Can you work these out from the model? Positions are in its coordinate system, mm. Face numbers are marked on the shaded views. A direction names the side the tool comes from. Round coordinates to 2 decimals unless told otherwise and drop trailing zeros. Order: outer loops, then holes, each group sorted by start corner. A loop starts at its lowest first (then second) coordinate and runs counter-clockwise, first axis right, second up. Notation, with made-up numbers: (68.5, 27) - (91.5, 27) arc R25 ccw to (91.5, 48) - close; hole circle Ø10 at (-22, 30.5). An arc over 180 degrees is marked (long way). Write item = value, one per line.
from build123d import *

# Parameters (mm, degrees)
P_IDAT_VYSUNUT_M1_DEPTH  = 8
SKICA2_W                 = 1.4
SKICA2_H                 = 2.8
ODEBRAT_VYSUNUT_M1_DEPTH = 4.4
SKICA3_W                 = 2
SKICA3_H                 = 2
P_IDAT_VYSUNUT_M2_DEPTH  = 4
P_IDAT_START             = 8
SKICA5_W                 = 16
SKICA5_H                 = 8
P_IDAT_VYSUNUT_M3_DEPTH  = 16
ODEBRAT_VYSUNUT_M3_DEPTH = 191.628493411
ODEBRAT_VYSUNUT_M4_DEPTH = 188.40870444
SKICA4_W                 = 2.8
SKICA4_H                 = 2.8
ODEBRAT_VYSUNUT_M2_DEPTH = 4.4
SKICA8_W                 = 1.4
SKICA8_H                 = 2.8
ODEBRAT_VYSUNUT_M5_DEPTH = 4.4


with BuildPart() as part:
    # Skica1 → Přidat vysunutím1 (new body)
    with BuildSketch(Plane(origin=(0, 0, 0), x_dir=(1, 0, 0), z_dir=(0, 1, 0))):
        Polygon((0, 0), (0, -111), (150.15, -55.45), (150.15, 0), (142.85, 0), (142.85, -50.153914462), (7.3, -100.30244926), (7.3, 0), align=None)
    extrude(amount=P_IDAT_VYSUNUT_M1_DEPTH)

    # Skica2 → Odebrat vysunutím1 (cut)
    with BuildSketch(Plane(origin=(0, 8, 0), x_dir=(1, 0, 0), z_dir=(0, 1, 0))):
        with Locations((0.7, -97)):
            Rectangle(SKICA2_W, SKICA2_H)
    extrude(amount=-ODEBRAT_VYSUNUT_M1_DEPTH, mode=Mode.SUBTRACT)

    # Skica3 → Přidat vysunutím2 (add)
    with BuildSketch(Plane.ZY):
        with Locations((6.3, 4)):
            Rectangle(SKICA3_W, SKICA3_H)
        with Locations((39.1, 4)):
            Rectangle(SKICA3_W, SKICA3_H)
        with Locations((71.9, 4)):
            Rectangle(SKICA3_W, SKICA3_H)
        with Locations((104.7, 4)):
            Rectangle(SKICA3_W, SKICA3_H)
    extrude(amount=P_IDAT_VYSUNUT_M2_DEPTH)

    # Skica5 → Přidat vysunutím3 (add)
    with BuildSketch(Plane(origin=(0, 8, 0), x_dir=(1, 0, 0), z_dir=(0, 1, 0)).offset(P_IDAT_START)):
        with Locations((8, -7)):
            Rectangle(SKICA5_W, SKICA5_H)
        with Locations((142.15, -7)):
            Rectangle(SKICA5_W, SKICA5_H)
    extrude(amount=-P_IDAT_VYSUNUT_M3_DEPTH)

    # Skica6 → Odebrat vysunutím3 (cut, through all)
    with BuildSketch(Plane(origin=(150.15, 0, 0), x_dir=(0, 0, -1), z_dir=(1, 0, 0))):
        Polygon((-11, 8), (-11, 16), (-3, 16), align=None)
    extrude(amount=-ODEBRAT_VYSUNUT_M3_DEPTH, mode=Mode.SUBTRACT)

    # Skica7 → Odebrat vysunutím4 (cut, through all)
    with BuildSketch(Plane.XZ):
        Polygon((7.3, 11), (16, 3), (16, 11), align=None)
        Polygon((134.15, 3), (134.15, 11), (142.85, 11), align=None)
    extrude(amount=-ODEBRAT_VYSUNUT_M4_DEPTH, mode=Mode.SUBTRACT)

    # Skica4 → Odebrat vysunutím2 (cut)
    with BuildSketch(Plane(origin=(150.15, 0, 0), x_dir=(0, 0, -1), z_dir=(1, 0, 0))):
        with Locations((-47, 4)):
            Rectangle(SKICA4_W, SKICA4_H)
        with Locations((-29.2, 4)):
            Rectangle(SKICA4_W, SKICA4_H)
        with Locations((-11.4, 4)):
            Rectangle(SKICA4_W, SKICA4_H)
    extrude(amount=-ODEBRAT_VYSUNUT_M2_DEPTH, mode=Mode.SUBTRACT)

    # Skica8 → Odebrat vysunutím5 (cut)
    with BuildSketch(Plane(origin=(0, 8, 0), x_dir=(1, 0, 0), z_dir=(0, 1, 0))):
        with Locations((149.45, -43)):
            Rectangle(SKICA8_W, SKICA8_H)
    extrude(amount=-ODEBRAT_VYSUNUT_M5_DEPTH, mode=Mode.SUBTRACT)


solid = part.part
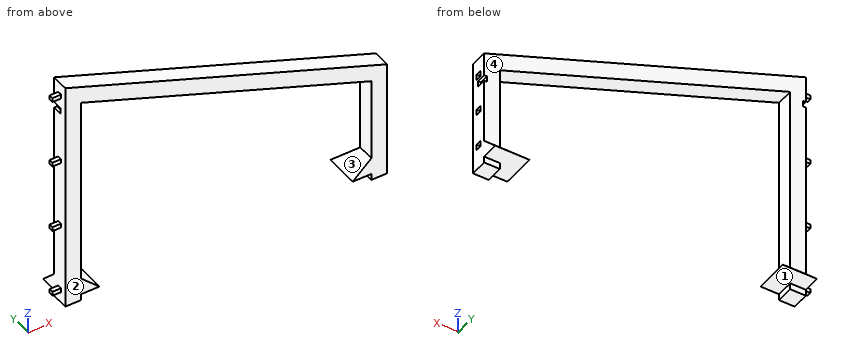
(1) Will these pins go through, and if not, where does the flat tip stop? P1, Ø2.5, axis at y = 5, z = 27, coming from the -X side; P2, Ø2, axis at x = -2.5, z = 6, coming from the -Y side; P3, Ø0.8, axis at x = 148, z = 11, coming from the +Y side.
Computed:
P1 = 0
P2 = 3
P3 = 8.4
(2) On a 3-axis mill with a long thin cutter (end or side, diameter ignored), from which of +Z, -Z, +X, -X, +Y, -Y can I reach the whole of each face in a straight line? I mean the marked faces 3 and 4. Say none if no direction works.
Computed:
face_3 = +Y, -Y
face_4 = +Z, +X, -X, +Y
(3) If we section it at A-A (z = 25): Write out the boundary of the cut face in (x, y).
Computed:
outline = (0, 0) - (7.3, 0) - (7.3, 8) - (0, 8) - close; (142.85, 0) - (150.15, 0) - (150.15, 8) - (142.85, 8) - close
(4) If we section it at B-B (x = 138.5): Write out the boundary of the cut face in (y, z).
Computed:
outline = (0, 3) - (16, 3) - (12, 7) - (0, 7) - close; (0, 51.76) - (8, 51.76) - (8, 59.76) - (0, 59.76) - close
(5) If we section it at C-C (x = 31): Write out the boundary of the cut face in (y, z), plus the area to 3 significant figures.
Computed:
outline = (0, 91.53) - (8, 91.53) - (8, 99.53) - (0, 99.53) - close
area = 64.0 mm^2
(6) Thinking about a two-plate mould opening in X: for the marked faces 1 and 2, which applies, +X half, -X half, draft (parallel to the pull), parting line (faces both ways), or undercut?
Computed:
face_1 = undercut
face_2 = draft
(7) If I drill on line 1 (X direction, y = 5.5, z = 20); line 2 (X direction, y = 5.75, z = 42.5); line 3 (Y direction, x = 8.5, z = 104), over which ranges is the centre line in solid material (lowest first)? Write a range as from..to.
Computed:
line_1 = 0..7.3, 142.85..150.15
line_2 = 0..7.3, 142.85..148.75
line_3 = 0..8
